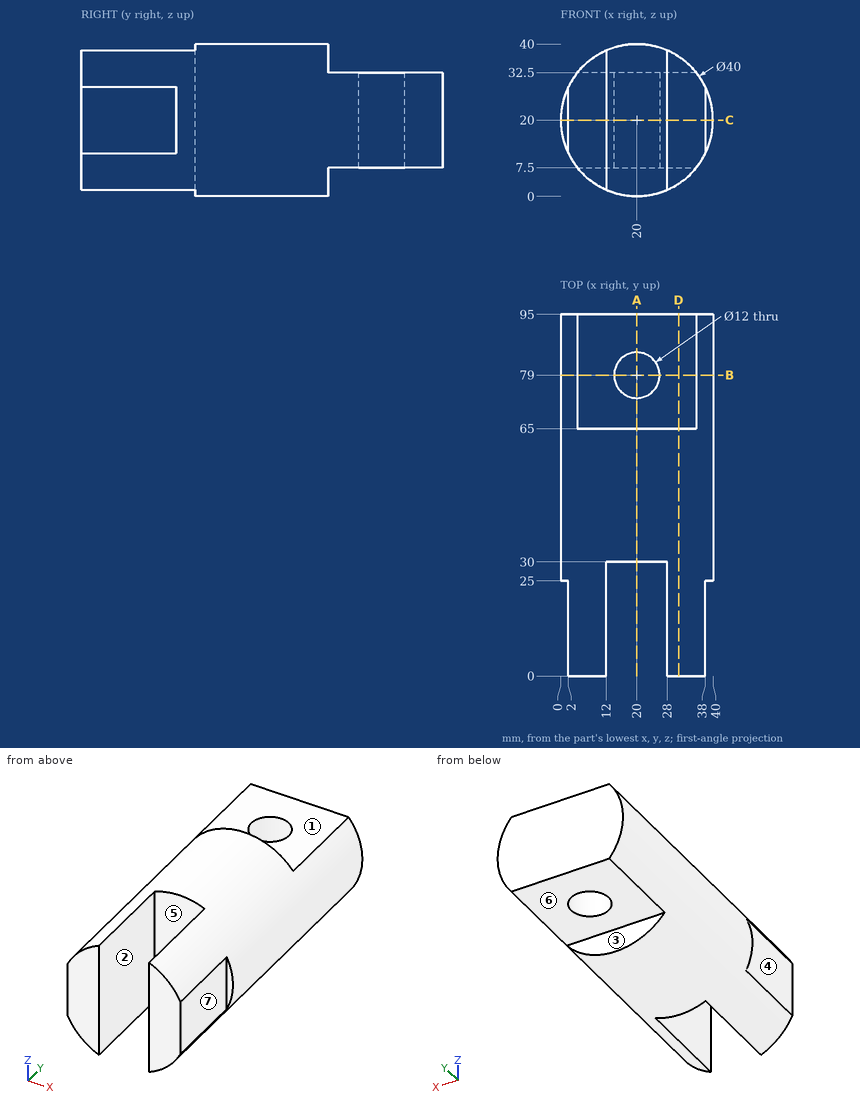
Check sheet for the drawn part. Datum: minimum x, y, z corner. Units: mm. A direction names the side the tool comes from. Round coordinates to 2 decimals unless told otherwise and drop trailing zeros. Order: outer loops, then holes, each group sorted by start corner. A loop starts at its lowest first (then second) coordinate and runs counter-clockwise, first axis right, second up. Notation, with made-up numbers: M -37,2.25 L 22,2.25 A22 cw 22,21.25 Z; hole C 13,10 d7. An arc over 180 degrees is marked long. Write each question's results on one line, items separated by ' | '. Start each with the question number.
1. Set-up check for the marked faces 1, 2, 3 and 4: record each of +Z, -Z, +X, -X, +Y, -Y from which the full face is reachable in a straight line by a thin tool's end or side.
2. Draft check along X on the marked faces 5, 6 and 7. Enter one of: pulls with the +X half, pulls with the -X half, needs draft (parallel to the pull), parting line crosses it, or undercut.
3. Go/stop test with flat-tipped pins: P1, Ø1.6, axis at x = 39, z = 20, coming from the -Y side; P2, Ø15, axis at x = 16, y = 84.5, coming from the +Z side; P3, Ø14, axis at y = 16.5, z = 17, coming from the -X side. Record where each tip stops, or that it passes through.
4. Cross-section at B-B on y = 79. Record the boundary of the cut face in (x, z).
5. Cross-section at C-C on z = 20. Record the boundary of the cut face in (x, y).
6. Cross-section at D-D on x = 31. Record the boundary of the cut face in (y, z).
7. Material ranges on L1, parallel to Y at x = 20, z = 21; L2, parallel to Y at x = 21, z = 34; L3, parallel to X at y = 63.5, z = 28, recorded low to high. Write a range as from..to.
8. Cross-section at A-A on x = 20. Record the boundary of the cut face in (y, z), plus the area to 3 significant figures.
Resolved:
1) face 1: +Z, +X, -X, +Y | face 2: +Z, -Z, -Y | face 3: -Z, +X, -X, +Y | face 4: +Z, -Z, -X, -Y
2) face 5: undercut | face 6: needs draft | face 7: pulls with the +X half
3) P1: y = 25 | P2: z = 32.5 | P3: x = 2
4) outline: M 4.39,7.5 L 14,7.5 L 14,32.5 L 4.39,32.5 A20 ccw Z; M 26,7.5 L 35.61,7.5 A20 ccw 35.61,32.5 L 26,32.5 Z
5) outline: M 0,25 L 2,25 L 2,0 L 12,0 L 12,30 L 28,30 L 28,0 L 38,0 L 38,25 L 40,25 L 40,95 L 0,95 Z; hole C 20,79 d12
6) outline: M 0,3.3 L 65,3.3 L 65,7.5 L 95,7.5 L 95,32.5 L 65,32.5 L 65,36.7 L 0,36.7 Z
7) L1: 30..73, 85..95 | L2: 30..65 | L3: 1.67..38.33
8) outline: M 30,0 L 65,0 L 65,7.5 L 73,7.5 L 73,32.5 L 65,32.5 L 65,40 L 30,40 Z; M 85,7.5 L 95,7.5 L 95,32.5 L 85,32.5 Z | area: 1,850 mm2
